```python
from build123d import *

# Parameters (mm, degrees)
SKETCH1_R           = 3.15
EXTRUDE1_DEPTH      = 1.5
SKETCH2_R           = 2.2051
EXTRUDE2_DEPTH      = 1.1
CHAMFER2_SIZE       = 0.127
SKETCH_2_R          = 2.6
EXTRUDE_1_DEPTH     = 2.6
SKETCH_1_R          = 1.25
CUT_EXTRUDE_1_DEPTH = 10
SKETCH_3_R          = 2.75
SKETCH_3_R_2        = 2.085
CUT_EXTRUDE_2_DEPTH = 1
CHAMFER_2_SIZE      = 0.1
CHAMFER_3_SIZE      = 0.3
CHAMFER_4_SIZE      = 0.3
SKETCH_6_R          = 1.25
EXTRUDE_2_DEPTH     = 3.2
HOLE_WIZARD_M31_D   = 2.5


with BuildPart() as part:
    # Sketch1 → Extrude1 (new body)
    with BuildSketch(Plane.XY):
        Circle(SKETCH1_R)
    extrude(amount=-EXTRUDE1_DEPTH)

    # Sketch2 → Extrude2 (add)
    with BuildSketch(Plane(origin=(0, 0, -1.5), x_dir=(-1, 0, 0), z_dir=(0, 0, -1))):
        with Locations(Location((0, 0, 0), (0, 0, 180))):
            Circle(SKETCH2_R)
    extrude(amount=EXTRUDE2_DEPTH)

    # Chamfer2
    chamfer2_edges = [part.edges().sort_by_distance(p)[0] for p in [
        (-3.15, 0, 0),
        (-3.15, 0, -1.5),
    ]]
    chamfer(chamfer2_edges, length=CHAMFER2_SIZE)

    # Эскиз2 → Бобышка-Вытянуть1 (add)
    with BuildSketch(Plane.XY):
        Circle(SKETCH_2_R)
    extrude(amount=-EXTRUDE_1_DEPTH)

    # Эскиз1 → Вырез-Вытянуть1 (cut)
    with BuildSketch(Plane.XY):
        Circle(SKETCH_1_R)
    extrude(amount=-CUT_EXTRUDE_1_DEPTH, mode=Mode.SUBTRACT)

    # Эскиз3 → Вырез-Вытянуть2 (cut)
    with BuildSketch(Plane(origin=(0, 0, -1.5), x_dir=(-1, 0, 0), z_dir=(0, 0, -1))):
        Circle(SKETCH_3_R)
        with Locations(Location((0, 0, 0), (0, 0, 90))):
            Circle(SKETCH_3_R_2, mode=Mode.SUBTRACT)
    extrude(amount=CUT_EXTRUDE_2_DEPTH, mode=Mode.SUBTRACT)

    # Фаска2
    chamfer_2_edges = [part.edges().sort_by_distance(p)[0] for p in [
        (0, -2.085, -2.5),
    ]]
    chamfer(chamfer_2_edges, length=CHAMFER_2_SIZE)

    # Фаска3
    # the kernel refuses this chamfer: 0.3 mm, written as the material it takes off along each edge
    with BuildSketch(Plane(origin=(0, 0, -2.6), x_dir=(1, 0, 0), z_dir=(0, -1, 0))) as chamfer_3_piece_1:
        Polygon((2.6, CHAMFER_3_SIZE), (2.6 - CHAMFER_3_SIZE, 0), (2.6, 0), align=None)
    revolve(axis=Axis((0, 0, -2.6), (0, 0, 1)), mode=Mode.SUBTRACT)

    # Фаска4
    chamfer_4_edges = [part.edges().sort_by_distance(p)[0] for p in [
        (-1.25, 0, -2.6),
    ]]
    chamfer(chamfer_4_edges, length=CHAMFER_4_SIZE)

    # Эскиз6 → Бобышка-Вытянуть2 (add)
    with BuildSketch(Plane.XY):
        Circle(SKETCH_6_R)
    extrude(amount=-EXTRUDE_2_DEPTH)

    # Отверстие обработанное метчиком M31 (through all)
    with Locations(Plane.XY):
        with Locations((0, 0)):
            Hole(HOLE_WIZARD_M31_D / 2)


solid = part.part
```
Model file for the job. Use its own axes, mm. A direction names the side the tool comes from. Coordinates: 2 decimals unless noted, no trailing zeros. Order: outer loops, then holes, each group sorted by start corner. A loop starts at its lowest first (then second) coordinate and runs counter-clockwise, first axis right, second up. Notation, with made-up numbers: (-19, 83.25) -> (17, 83.25) arc R27 ccw to (17, 121.25) -> close; hole circle Ø3 at (-3.5, 43.5). An arc over 180 degrees is marked (long way). Answer as a JSON object with one key per item and string values. Group by question number.
1) Drill centre lines: L1, parallel to Y at x = 0, z = -0.5; L2, parallel to X at y = 0, z = -1.8 (3 decimals); L3, parallel to Z at x = -2.5, y = -0.75. Where is each one in solid material? Low to high.
2) Cut at C-C, the plane z = -1.7. Write the cut outline in (x, y) (3 decimals).
3) Flat gauge pins, fed straight in: pin 1 (1.5 mm diameter, centred on x = -0.5, y = 2.5, fed in from +Z); pin 2 (1.5 mm diameter, centred on x = 0, y = 0, fed in from +Z); pin 3 (1 mm diameter, centred on x = -1, z = -0.5, fed in from +Y). Where does each tip first touch, or does it go through?
4) Pull direction Y, two halves, no side cores. Call faces 1 (the face through (2, 0, -2.6)), 2 (the face through (0.27, -1.22, -1.17)), 3 (the face through (-2.5, -1.917, -0.741)): +Y half, -Y half, draft (parallel to the pull), parting line (faces both ways), or undercut.
5) Which spindle directions (+Z, -Z, +X, -X, +Y, -Y) get a long thin tool onto all of the face, cutting with end or side? Do faces 4 (the face through (1, -1, 0)), 5 (the face through (-2.035, -0.452, -1.944)). Say none if no direction does.
6) Cut at D-D, the plane z = -0.7. Write the cut outline in (x, y).
7) Cut at A-A, the plane y = 0. Write the cut outline in (x, z) (3 decimals), then the cut area to 3 significant figures.
Check values:
{
 "1": {"L1": "y = -3.15 to -1.25, 1.25 to 3.15", "L2": "x = -2.085 to -1.25, 1.25 to 2.085", "L3": "z = -1.5 to 0"},
 "2": {"outline": "circle Ø4.17 at (0, 0); hole circle Ø2.5 at (0, 0)"},
 "3": {"pin 1": "stops at z = 0", "pin 2": "passes through", "pin 3": "stops at y = 3.11"},
 "4": {"face 1": "draft", "face 2": "undercut", "face 3": "parting line"},
 "5": {"face 4": "+Z, +X, -X, +Y, -Y", "face 5": "none"},
 "6": {"outline": "circle Ø6.3 at (0, 0); hole circle Ø2.5 at (0, 0)"},
 "7": {"outline": "(-3.15, -1.373) -> (-3.023, -1.5) -> (-2.085, -1.5) -> (-2.085, -2.4) -> (-2.185, -2.5) -> (-2.4, -2.5) -> (-2.3, -2.6) -> (-1.55, -2.6) -> (-1.25, -2.3) -> (-1.25, 0) -> (-3.023, 0) -> (-3.15, -0.127) -> close; (1.25, -2.3) -> (1.55, -2.6) -> (2.3, -2.6) -> (2.4, -2.5) -> (2.185, -2.5) -> (2.085, -2.4) -> (2.085, -1.5) -> (3.023, -1.5) -> (3.15, -1.373) -> (3.15, -0.127) -> (3.023, 0) -> (1.25, 0) -> close", "area": "7.48 mm²"}
}
